Model file for the job. Use its own axes, mm. A direction names the side the tool comes from. Round coordinates to 2 decimals unless told otherwise and drop trailing zeros. Use a Markdown table: item, result.
from build123d import *

# Parameters (mm, degrees)
F0_R     = 5.25
F1_DEPTH = 10
F0_R_2   = 60.5
F2_DEPTH = 8
F3_SIZE  = 1
F0_R_3   = 3.5
F4_DEPTH = 3


with BuildPart() as f1:
    # F0 (on Top) → F1 (new body)
    with BuildSketch(Plane.XY):
        with BuildLine():
            ThreePointArc((7.5, 49.4342998332), (37.9143772203, 32.596012026), (50, 0))
            ThreePointArc((50, 0), (49.1328198544, -9.2717858665), (46.5613594739, -18.2219593882))
            Line((46.5613594739, -18.2219593882), (53.7760869447, -22.3873842357))
            ThreePointArc((53.7760869447, -22.3873842357), (57.1205723209, -11.4150215828), (58.25, 0))
            ThreePointArc((58.25, 0), (43.7603559172, 38.4459848359), (7.5, 57.7651495281))
            Line((7.5, 57.7651495281), (7.5, 49.4342998332))
        make_face()
        with BuildLine():
            ThreePointArc((0, 50), (3.7606520937, 49.8583743801), (7.5, 49.4342998332))
            Line((7.5, 49.4342998332), (7.5, 57.7651495281))
            Line((7.5, 57.7651495281), (-7.5, 57.7651495281))
            Line((-7.5, 57.7651495281), (-7.5, 49.4342998332))
            ThreePointArc((-7.5, 49.4342998332), (-3.7606520937, 49.8583743801), (0, 50))
        make_face()
        with BuildLine():
            ThreePointArc((-46.5613594739, -18.2219593882), (-43.3012701892, 25), (-7.5, 49.4342998332))
            Line((-7.5, 49.4342998332), (-7.5, 57.7651495281))
            ThreePointArc((-7.5, 57.7651495281), (-50.4459797704, 29.125), (-53.7760869447, -22.3873842357))
            Line((-53.7760869447, -22.3873842357), (-46.5613594739, -18.2219593882))
        make_face()
        with BuildLine():
            Line((-46.2760869447, -35.3777652924), (-39.0613594739, -31.212340445))
            ThreePointArc((-39.0613594739, -31.212340445), (-43.3012701892, -25), (-46.5613594739, -18.2219593882))
            Line((-46.5613594739, -18.2219593882), (-53.7760869447, -22.3873842357))
            ThreePointArc((-53.7760869447, -22.3873842357), (-50.4459797704, -29.125), (-46.2760869447, -35.3777652924))
        make_face()
        with BuildLine():
            Line((46.2760869447, -35.3777652924), (39.0613594739, -31.212340445))
            ThreePointArc((39.0613594739, -31.212340445), (0, -50), (-39.0613594739, -31.212340445))
            Line((-39.0613594739, -31.212340445), (-46.2760869447, -35.3777652924))
            ThreePointArc((-46.2760869447, -35.3777652924), (0, -58.25), (46.2760869447, -35.3777652924))
        make_face()
        with BuildLine():
            Line((53.7760869447, -22.3873842357), (46.5613594739, -18.2219593882))
            ThreePointArc((46.5613594739, -18.2219593882), (43.3012701892, -25), (39.0613594739, -31.212340445))
            Line((39.0613594739, -31.212340445), (46.2760869447, -35.3777652924))
            ThreePointArc((46.2760869447, -35.3777652924), (50.4459797704, -29.125), (53.7760869447, -22.3873842357))
        make_face()
        with BuildLine():
            Line((-7.5, 57.7651495281), (7.5, 57.7651495281))
            ThreePointArc((7.5, 57.7651495281), (0, 58.25), (-7.5, 57.7651495281))
        make_face()
        with BuildLine():
            Line((7.5, 40), (7.5, 49.4342998332))
            ThreePointArc((7.5, 49.4342998332), (3.7606520937, 49.8583743801), (0, 50))
            Line((0, 50), (0, 47.5))
            ThreePointArc((0, 47.5), (5.3033008589, 45.3033008589), (7.5, 40))
        make_face()
        with BuildLine():
            Line((0, 47.5), (0, 50))
            ThreePointArc((0, 50), (-3.7606520937, 49.8583743801), (-7.5, 49.4342998332))
            Line((-7.5, 49.4342998332), (-7.5, 40))
            ThreePointArc((-7.5, 40), (-5.3033008589, 45.3033008589), (0, 47.5))
        make_face()
        with BuildLine():
            ThreePointArc((-7.5, 40), (0, 32.5), (7.5, 40))
            ThreePointArc((7.5, 40), (5.3033008589, 45.3033008589), (0, 47.5))
            ThreePointArc((0, 47.5), (-5.3033008589, 45.3033008589), (-7.5, 40))
        make_face()
        with BuildLine():
            ThreePointArc((5.25, 40), (-3.7123106012, 36.2876893988), (0, 45.25))
            ThreePointArc((0, 45.25), (3.7123106012, 43.7123106012), (5.25, 40))
        make_face(mode=Mode.SUBTRACT)
        with BuildLine():
            ThreePointArc((39.0613594739, -31.212340445), (43.3012701892, -25), (46.5613594739, -18.2219593882))
            Line((46.5613594739, -18.2219593882), (38.3910161948, -13.5048094967))
            ThreePointArc((38.3910161948, -13.5048094967), (41.1362066923, -16.2500000217), (42.1410161514, -20))
            ThreePointArc((42.1410161514, -20), (38.3910161049, -26.4951905552), (30.8910160584, -26.4951904747))
            Line((30.8910160584, -26.4951904747), (39.0613594739, -31.212340445))
        make_face()
        with BuildLine():
            ThreePointArc((42.1410161514, -20), (41.1362066923, -16.2500000217), (38.3910161948, -13.5048094967))
            ThreePointArc((38.3910161948, -13.5048094967), (28.1458256624, -16.2499999318), (30.8910160584, -26.4951904747))
            ThreePointArc((30.8910160584, -26.4951904747), (38.3910161049, -26.4951905552), (42.1410161514, -20))
        make_face()
        with Locations((34.6410161514, -20)):
            Circle(F0_R, mode=Mode.SUBTRACT)
        with BuildLine():
            ThreePointArc((-38.3910159202, -13.5048093381), (-41.1362067455, -23.7499998861), (-30.891016148, -26.4951905264))
            ThreePointArc((-30.891016148, -26.4951905264), (-28.145825622, -23.7499999983), (-27.1410161514, -20))
            ThreePointArc((-27.1410161514, -20), (-30.8910160358, -13.5048095384), (-38.3910159202, -13.5048093381))
        make_face()
        with Locations((-34.6410161514, -20)):
            Circle(F0_R, mode=Mode.SUBTRACT)
        with BuildLine():
            ThreePointArc((-46.5613594739, -18.2219593882), (-43.3012701892, -25), (-39.0613594739, -31.212340445))
            Line((-39.0613594739, -31.212340445), (-30.891016148, -26.4951905264))
            ThreePointArc((-30.891016148, -26.4951905264), (-41.1362067455, -23.7499998861), (-38.3910159202, -13.5048093381))
            Line((-38.3910159202, -13.5048093381), (-46.5613594739, -18.2219593882))
        make_face()
    extrude(amount=F1_DEPTH)

    # F0 (on Top) → F2 (join)
    with BuildSketch(Plane.XY):
        Circle(F0_R_2)
        with BuildLine():
            ThreePointArc((-7.5, 57.7651495281), (0, 58.25), (7.5, 57.7651495281))
            ThreePointArc((7.5, 57.7651495281), (43.7603559172, 38.4459848359), (58.25, 0))
            ThreePointArc((58.25, 0), (57.1205723209, -11.4150215828), (53.7760869447, -22.3873842357))
            ThreePointArc((53.7760869447, -22.3873842357), (50.4459797704, -29.125), (46.2760869447, -35.3777652924))
            ThreePointArc((46.2760869447, -35.3777652924), (0, -58.25), (-46.2760869447, -35.3777652924))
            ThreePointArc((-46.2760869447, -35.3777652924), (-50.4459797704, -29.125), (-53.7760869447, -22.3873842357))
            ThreePointArc((-53.7760869447, -22.3873842357), (-50.4459797704, 29.125), (-7.5, 57.7651495281))
        make_face(mode=Mode.SUBTRACT)
    extrude(amount=F2_DEPTH)

    # F3
    f3_edges = [f1.edges().sort_by_distance(p)[0] for p in [
        (-7.5, -57.76515, 10),
    ]]
    chamfer(f3_edges, length=F3_SIZE)

    # F0 (on Top) → F4 (join)
    with BuildSketch(Plane.XY):
        with BuildLine():
            ThreePointArc((5.25, 40), (3.7123106012, 43.7123106012), (0, 45.25))
            ThreePointArc((0, 45.25), (-3.7123106012, 36.2876893988), (5.25, 40))
        make_face()
        with BuildLine():
            ThreePointArc((3.5, 40), (-2.4748737342, 37.5251262658), (0, 43.5))
            ThreePointArc((0, 43.5), (2.4748737342, 42.4748737342), (3.5, 40))
        make_face(mode=Mode.SUBTRACT)
        with Locations((-34.6410161514, -20)):
            Circle(F0_R)
        with Locations((-34.6410161514, -20)):
            Circle(F0_R_3, mode=Mode.SUBTRACT)
        with Locations((34.6410161514, -20)):
            Circle(F0_R)
        with Locations((34.6410161514, -20)):
            Circle(F0_R_3, mode=Mode.SUBTRACT)
    extrude(amount=F4_DEPTH)


solid = f1.part
Q1. Flat gauge pins, fed straight in: pin 1 (4 mm diameter, centred on x = 34.64, y = -20, fed in from -Z); pin 2 (3 mm diameter, centred on x = -23.5, z = 2, fed in from +Y); pin 3 (5 mm diameter, centred on y = 6.5, z = 3.5, fed in from +X); pin 4 (1.5 mm diameter, centred on y = -21.5, z = 2.5, fed in from -X). Where does each tip first touch, or does it go through?
Results list:
| item | result |
|---|---|
| pin 1 | passes through |
| pin 2 | stops at y = 56.36 |
| pin 3 | stops at x = 60.37 |
| pin 4 | stops at x = -56.83 |
Q2. Band-saw the part on A-A, the plane x = 2. Give the number of separate pieces and of enclosed holes in the cut face, plus the area to 3 significant figures.
Results list:
| item | result |
|---|---|
| separate pieces | 3 |
| enclosed holes | 0 |
| area | 287 mm² |
Q3. Tool access for faces 5 (the face through (-4, 40, 3)), 6 (the face through (-35.033, -28.887, 4.93)), 7 (the face through (-5, 36, 0)): list every direction of +Z, -Z, +X, -X, +Y, -Y with a clear straight run to the whole face (end or side of a thin tool).
Results list:
| item | result |
|---|---|
| face 5 | +Z |
| face 6 | +Z, -Z |
| face 7 | -Z, +X, -X, +Y, -Y |
Q4. Pull direction X, two halves, no side cores. Call faces 1 (the face through (-13.12, -59.06, 3.94)), 2 (the face through (-32, 50, 8)), 3 (the face through (28.23, -16.11, 4.93)), 4 (the face through (-0.16, 32.5, 4.93)): released by +X, released by -X, zero draft, split by the parting line, or undercut.
Results list:
| item | result |
|---|---|
| face 1 | split by the parting line |
| face 2 | zero draft |
| face 3 | undercut |
| face 4 | undercut |
Q5. Drill centre lines: L1, parallel to X at y = -21.5, z = 8.75; L2, parallel to X at y = 45.5, z = 3; L3, parallel to Y at x = 28.5, z = 4.25. Where is each one in solid material? Low to high. Write a range as from..to.
Results list:
| item | result |
|---|---|
| L1 | x = -54.14..-39.67, -29.61..-27.29, 27.29..29.61, 39.67..54.14 |
| L2 | x = -39.87..-20.73, -7.5..7.5, 20.73..39.87 |
| L3 | y = -53.37..-41.08, -24.31..-15.69, 41.08..53.37 |
